Design review of the part shown in the three views and the two pictorial views. Dimensions are in mm from the part's minimum x, y and z. A direction names the side the tool comes from. Coordinates: 2 decimals unless noted, no trailing zeros. Loops run counter-clockwise (first coordinate to the right, second up) from the corner with the lowest first, then second, coordinate; pieces in that order, holes last. Notation, with made-up numbers: (36.5, -9) -> (70.5, -9) arc R10 ccw to (70.5, 8) -> close; hole circle Ø2 at (71, -31.5). An arc over 180 degrees is marked (long way). One line per item, written item: value. Start each with the question number.
1. Draft analysis for pull direction X (two halves, no side actions). For the marked faces 3, 4, 5 and 6, state which applies: pulls with the +X half, pulls with the -X half, needs draft (parallel to the pull), parting line crosses it, or undercut.
2. Insertion check: pin 1 (6 mm diameter, centred on y = 6, z = 92, fed in from +X); pin 2 (8 mm diameter, centred on x = 67, z = 19, fed in from -Y). Each pin has a flat end and moves straight along its axis. Give the tip position at first contact, or say it passes through.
3. Add section B-B on y = 11. Write out the cut boundary in (x, z), plus the area to 3 significant figures.
4. Add section D-D on y = 2.75. Write out the cut boundary in (x, z).
5. Add section C-C on x = 26. Write out the cut boundary in (y, z).
6. For probe 1 along Z at (x, y) = (35, 9); probe 2 along Y at (x, z) = (103, 22), list the stretches that pass through material, from the lowest coordinate up.
7. Add section A-A on z = 2.5. Write out the cut boundary in (x, y).
8. Machinability: for the marked faces 1 and 2, which of the approach directions +Z, -Z, +X, -X, +Y, -Y give a long, thin tool a straight path to every point of the face, cutting with its end or side? Answer none if there is none.
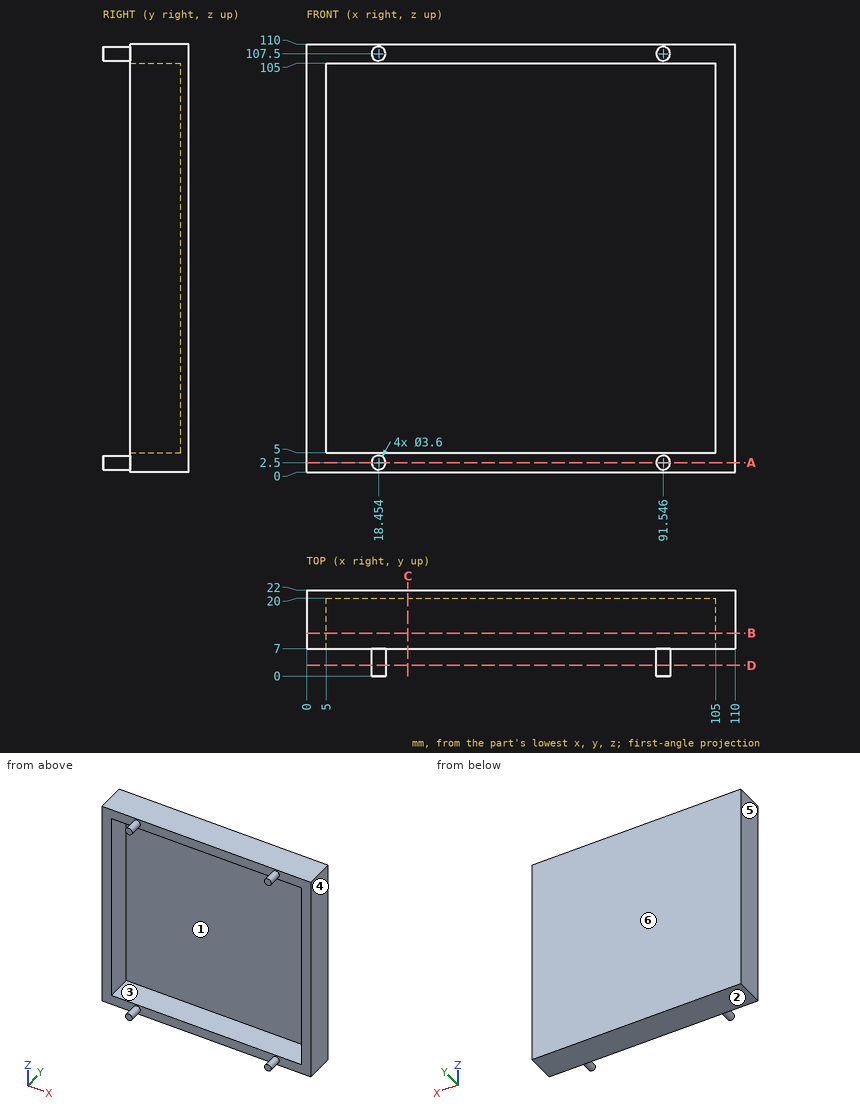
Worked answers:
1. face 3: undercut
1. face 4: pulls with the +X half
1. face 5: pulls with the -X half
1. face 6: needs draft
2. pin 1: stops at x = 110
2. pin 2: stops at y = 20
3. outline: (0, 0) -> (110, 0) -> (110, 110) -> (0, 110) -> close; hole (5, 5) -> (105, 5) -> (105, 105) -> (5, 105) -> close
3. area: 2,100 mm²
4. outline: circle Ø3.6 at (18.45, 2.5); circle Ø3.6 at (18.45, 107.5); circle Ø3.6 at (91.55, 2.5); circle Ø3.6 at (91.55, 107.5)
5. outline: (7, 0) -> (22, 0) -> (22, 110) -> (7, 110) -> (7, 105) -> (20, 105) -> (20, 5) -> (7, 5) -> close
6. probe 1: z = 0 to 5, 105 to 110
6. probe 2: y = 20 to 22
7. outline: (0, 7) -> (16.65, 7) -> (16.65, 0) -> (20.25, 0) -> (20.25, 7) -> (89.75, 7) -> (89.75, 0) -> (93.35, 0) -> (93.35, 7) -> (110, 7) -> (110, 22) -> (0, 22) -> close
8. face 1: -Y
8. face 2: -Z, +X, -X, +Y, -Y
